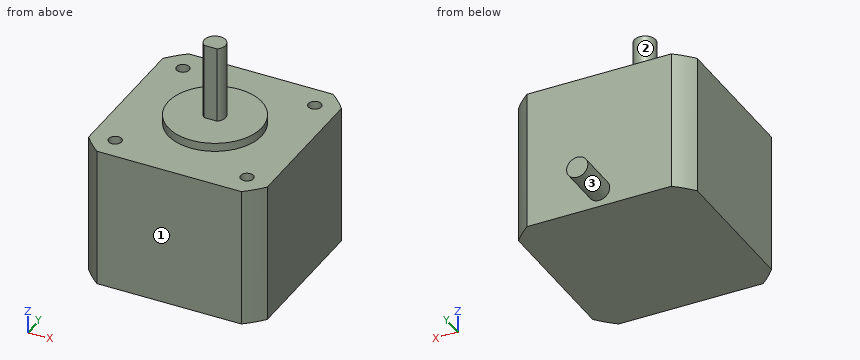
```python
from build123d import *

# Parameters (mm, degrees)
SKETCH_1_W                   = 42
SKETCH_1_H                   = 42
EXTRUDE_1_DEPTH              = 33
SKETCH_2_R                   = 11
EXTRUDE_2_DEPTH              = 2
SKETCH_3_R                   = 2.5
EXTRUDE_3_DEPTH              = 18
CUT_EXTRUDE_2_DEPTH          = 18
HOLE_WIZARD_M3_1_D           = 2.5
HOLE_WIZARD_M3_1_DEPTH       = 7.5
HOLE_WIZARD_M3_1_CBORE_D     = 3
HOLE_WIZARD_M3_1_CBORE_DEPTH = 6
HOLE_WIZARD_M3_1_TIP         = 0.751075774
SKETCH_7_OUTSIDE_W           = 59.922
SKETCH_7_OUTSIDE_H           = 59.922
SKETCH_7_OUTSIDE_R           = 27
CUT_EXTRUDE_3_DEPTH          = 34
SKETCH_8_R                   = 2.5
EXTRUDE_4_DEPTH              = 10


with BuildPart() as part:
    # 草圖1 → 填料-伸長1 (new body)
    with BuildSketch(Plane.XY):
        Rectangle(SKETCH_1_W, SKETCH_1_H)
    extrude(amount=-EXTRUDE_1_DEPTH)

    # 草圖2 → 填料-伸長2 (add)
    with BuildSketch(Plane.XY):
        Circle(SKETCH_2_R)
    extrude(amount=EXTRUDE_2_DEPTH)

    # 草圖3 → 填料-伸長3 (add)
    with BuildSketch(Plane.XY.offset(2)):
        Circle(SKETCH_3_R)
    extrude(amount=EXTRUDE_3_DEPTH)

    # 草圖4 → 除料-伸長2 (cut)
    with BuildSketch(Plane.XY.offset(20)):
        with BuildLine():
            Line((1.5, -2), (-1.5, -2))
            ThreePointArc((-1.5, -2), (0, -2.5), (1.5, -2))
        make_face()
    extrude(amount=-CUT_EXTRUDE_2_DEPTH, mode=Mode.SUBTRACT)

    # M3 螺紋孔1
    with Locations(Plane.XY):
        with Locations((-15.5, 15.5), (15.5, 15.5), (15.5, -15.5), (-15.5, -15.5)):
            CounterBoreHole(HOLE_WIZARD_M3_1_D / 2, HOLE_WIZARD_M3_1_CBORE_D / 2, HOLE_WIZARD_M3_1_CBORE_DEPTH, depth=HOLE_WIZARD_M3_1_DEPTH)
            with Locations((0, 0, -(HOLE_WIZARD_M3_1_DEPTH + HOLE_WIZARD_M3_1_TIP / 2))):  # 118° drill point
                Cone(0, HOLE_WIZARD_M3_1_D / 2, HOLE_WIZARD_M3_1_TIP, mode=Mode.SUBTRACT)

    # 草圖7 outside → 除料-伸長3 (cut, through all)
    with BuildSketch(Plane.XY):
        Rectangle(SKETCH_7_OUTSIDE_W, SKETCH_7_OUTSIDE_H)
        Circle(SKETCH_7_OUTSIDE_R, mode=Mode.SUBTRACT)
    extrude(amount=-CUT_EXTRUDE_3_DEPTH, mode=Mode.SUBTRACT)

    # 草圖8 → 填料-伸長4 (add)
    with BuildSketch(Plane(origin=(0, 21, 0), x_dir=(1, 0, 0), z_dir=(0, 1, 0))):
        with Locations((0, 29)):
            Circle(SKETCH_8_R)
    extrude(amount=EXTRUDE_4_DEPTH)


solid = part.part
```
Geometry check sheet. Reference: the model listing, model coordinates, mm. Face numbers are marked on the shaded views. A direction names the side the tool comes from. Round coordinates to 2 decimals unless told otherwise and drop trailing zeros. Order: outer loops, then holes, each group sorted by start corner. A loop starts at its lowest first (then second) coordinate and runs counter-clockwise, first axis right, second up. Notation, with made-up numbers: (76.5, -12.5) - (85.5, -12.5) arc R15 ccw to (85.5, 14.5) - close; hole circle Ø7 at (-17.75, -15). An arc over 180 degrees is marked (long way). Use a Markdown table: item, result. Add a question column.
1) Section check D-D (z = -29). Record the cut outline in (x, y), then the cut area to 3 significant figures.
2) Section check C-C (x = 10). Record the cut outline in (y, z).
3) Thickness scan on line 1 along Y through (x, z) = (15.5, -7.1); line 2 along X through (y, z) = (15, -4). Record the ranges inside material, lowest first.
4) Section check A-A (y = 0). Record the cut outline in (x, z), then the cut area to 3 significant figures.
5) Set-up check for the marked faces 1, 2 and 3: record each of +Z, -Z, +X, -X, +Y, -Y from which the full face is reachable in a straight line by a thin tool's end or side.
6) Gauge pin test, flat ends, axial feed: P1, Ø5, axis at x = 6, y = -12.5, coming from the +Z side; P2, Ø1.5, axis at x = 16, y = 15, coming from the +Z side; P3, Ø10, axis at x = -5.5, z = -11, coming from the +Y side. Record the tip position at first contact, or that the pin passes through.
7) Section check B-B (z = -23.5). Record the cut outline in (x, y), then the cut area to 3 significant figures.
Established:
| question | item | result |
|---|---|---|
| 1 | outline | (-21, -16.97) arc R27 ccw to (-16.97, -21) - (16.97, -21) arc R27 ccw to (21, -16.97) - (21, 16.97) arc R27 ccw to (16.97, 21) - (2.5, 21) - (2.5, 31) - (-2.5, 31) - (-2.5, 21) - (-16.97, 21) arc R27 ccw to (-21, 16.97) - close |
| 1 | area | 1,780 mm2 |
| 2 | outline | (-21, -33) - (21, -33) - (21, 0) - (4.58, 0) - (4.58, 2) - (-4.58, 2) - (-4.58, 0) - (-21, 0) - close |
| 3 | line 1 | -21 to -16.75, -14.25 to 14.25, 16.75 to 21 |
| 3 | line 2 | -21 to -16.91, -14.09 to 14.09, 16.91 to 21 |
| 4 | outline | (-21, -33) - (21, -33) - (21, 0) - (11, 0) - (11, 2) - (2.5, 2) - (2.5, 20) - (-2.5, 20) - (-2.5, 2) - (-11, 2) - (-11, 0) - (-21, 0) - close |
| 4 | area | 1,520 mm2 |
| 5 | face 1 | +Z, -Z, +X, -X, -Y |
| 5 | face 2 | +Z |
| 5 | face 3 | +Y |
| 6 | P1 | z = 0 |
| 6 | P2 | z = -6 |
| 6 | P3 | y = 21 |
| 7 | outline | (-21, -16.97) arc R27 ccw to (-16.97, -21) - (16.97, -21) arc R27 ccw to (21, -16.97) - (21, 16.97) arc R27 ccw to (16.97, 21) - (-16.97, 21) arc R27 ccw to (-21, 16.97) - close |
| 7 | area | 1,730 mm2 |
